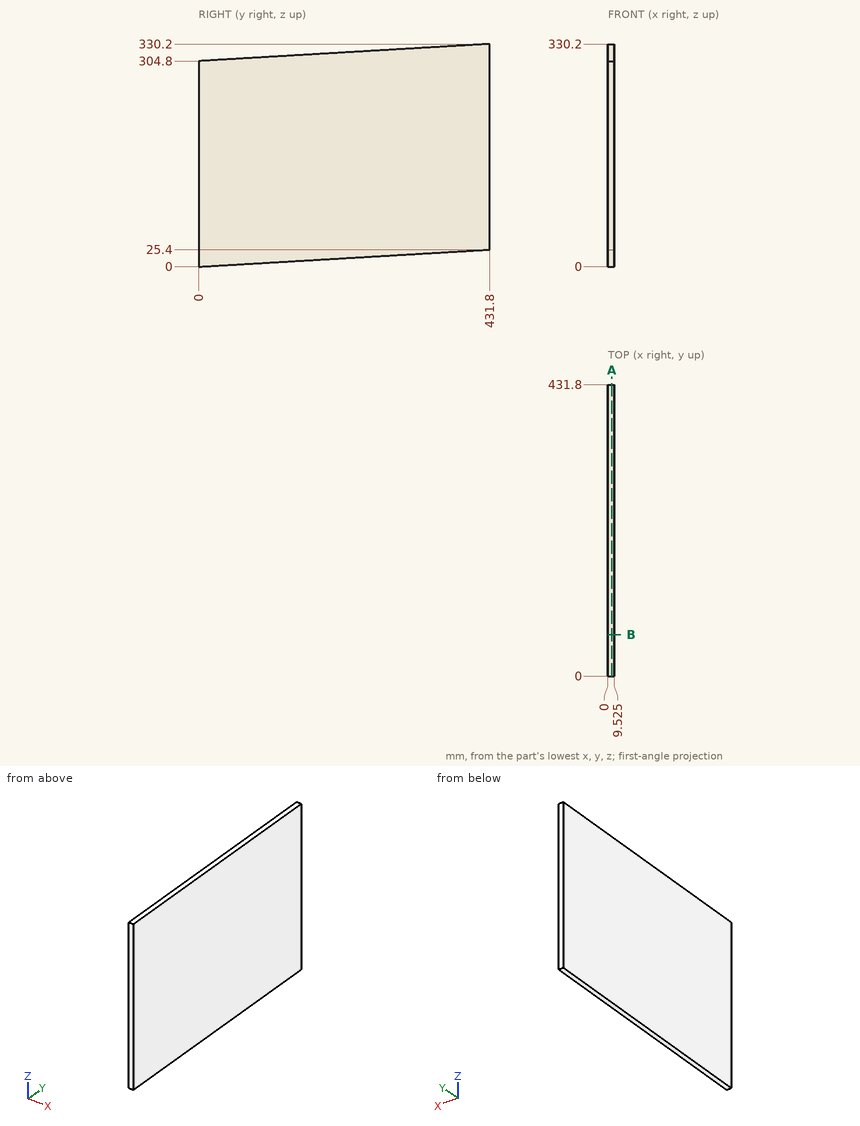
The drawing under review shows one solid part. Ordinate dimensions are in mm from its lowest x, y, z. Round coordinates to 2 decimals unless told otherwise and drop trailing zeros. Order: outer loops, then holes, each group sorted by start corner. A loop starts at its lowest first (then second) coordinate and runs counter-clockwise, first axis right, second up. Notation, with made-up numbers: (11.5, 4) -> (32.5, 4) arc R23 ccw to (32.5, 22) -> close; hole circle Ø6 at (20, -31.75). An arc over 180 degrees is marked (long way). Use a Markdown table: item, result.
Q1. For line 1 (Z direction, x = 8.25, y = 297.5); line 2 (Z direction, x = 1.5, y = 100), list the stretches that pass through material, from the lowest coordinate up.
Values:
| item | result |
|---|---|
| line 1 | z = 17.5 to 322.3 |
| line 2 | z = 5.88 to 310.68 |
Q2. We need section B-B on y = 61.5. Write out the cut boundary in (x, z) (3 decimals).
Values:
| item | result |
|---|---|
| outline | (0, 3.618) -> (9.525, 3.618) -> (9.525, 308.418) -> (0, 308.418) -> close |
Q3. We need section A-A on x = 5.75. Write out the cut boundary in (y, z), then the cut area to 3 significant figures.
Values:
| item | result |
|---|---|
| outline | (0, 0) -> (431.8, 25.4) -> (431.8, 330.2) -> (0, 304.8) -> close |
| area | 132,000 mm^2 |
